The listing builds one solid part. Answer for the finished solid, in the listing's coordinates (mm). A direction names the side the tool comes from. Coordinates: 2 decimals unless noted, no trailing zeros. Write each loop counter-clockwise with the first axis right and the second up, starting at its lowest first coordinate (ties: lowest second). Pieces come first, ordered by that corner, then holes. Notation, with made-up numbers: M 59.25,-18 L 74.25,-18 A25 ccw 74.25,14 Z; hole C 85,42 d2. An arc over 180 degrees is marked long. Answer as CSV lines item,"result".
```python
from build123d import *

# Parameters (mm, degrees)
SKETCH1_W           = 15.307395447
SKETCH1_H           = 3.175
BOSS_EXTRUDE1_DEPTH = 16.27
SKETCH3_R           = 15.307395447
BOSS_EXTRUDE2_DEPTH = 3.175
CUT_EXTRUDE1_DEPTH  = 23.62
FILLET1_R           = 0.42


with BuildPart() as part:
    # Sketch1 → Revolve1 (revolve)
    with BuildSketch(Plane.XZ):
        with Locations((7.653697724, 1.5875)):
            Rectangle(SKETCH1_W, SKETCH1_H)
    revolve(axis=Axis((0, 0, 3.175), (0, 0, -1)))

    # Sketch2 → Boss-Extrude1 (add)
    with BuildSketch(Plane.XY.offset(3.175)):
        with BuildLine():
            Line((1.563453637, -12.031235681), (1.477576398, -11.370385062))
            ThreePointArc((1.477576398, -11.370385062), (0, -10.072395447), (-1.477576398, -11.370385062))
            Line((-1.477576398, -11.370385062), (-1.563453637, -12.031235681))
            ThreePointArc((-1.563453637, -12.031235681), (-2.366912935, -11.899274871), (-3.159711751, -11.713720201))
            Line((-3.159711751, -11.713720201), (-2.986155391, -11.070310044))
            ThreePointArc((-2.986155391, -11.070310044), (-3.854538862, -9.305679997), (-5.716360575, -9.939422028))
            Line((-5.716360575, -9.939422028), (-6.048597381, -10.517104592))
            ThreePointArc((-6.048597381, -10.517104592), (-6.740397766, -10.087718139), (-7.401839667, -9.612897005))
            Line((-7.401839667, -9.612897005), (-6.995272092, -9.084880673))
            ThreePointArc((-6.995272092, -9.084880673), (-7.122259124, -7.122259124), (-9.084880673, -6.995272092))
            Line((-9.084880673, -6.995272092), (-9.612897005, -7.401839667))
            ThreePointArc((-9.612897005, -7.401839667), (-10.087718139, -6.740397766), (-10.517104592, -6.048597381))
            Line((-10.517104592, -6.048597381), (-9.939422028, -5.716360575))
            ThreePointArc((-9.939422028, -5.716360575), (-9.305679997, -3.854538862), (-11.070310044, -2.986155391))
            Line((-11.070310044, -2.986155391), (-11.713720201, -3.159711751))
            ThreePointArc((-11.713720201, -3.159711751), (-11.899274871, -2.366912935), (-12.031235681, -1.563453637))
            Line((-12.031235681, -1.563453637), (-11.370385062, -1.477576398))
            ThreePointArc((-11.370385062, -1.477576398), (-10.072395447, 0), (-11.370385062, 1.477576398))
            Line((-11.370385062, 1.477576398), (-12.031235681, 1.563453637))
            ThreePointArc((-12.031235681, 1.563453637), (-11.899274871, 2.366912935), (-11.713720201, 3.159711751))
            Line((-11.713720201, 3.159711751), (-11.070310044, 2.986155391))
            ThreePointArc((-11.070310044, 2.986155391), (-9.305679997, 3.854538862), (-9.939422028, 5.716360575))
            Line((-9.939422028, 5.716360575), (-10.517104592, 6.048597381))
            ThreePointArc((-10.517104592, 6.048597381), (-10.087718139, 6.740397766), (-9.612897005, 7.401839667))
            Line((-9.612897005, 7.401839667), (-9.084880673, 6.995272092))
            ThreePointArc((-9.084880673, 6.995272092), (-7.122259124, 7.122259124), (-6.995272092, 9.084880673))
            Line((-6.995272092, 9.084880673), (-7.401839667, 9.612897005))
            ThreePointArc((-7.401839667, 9.612897005), (-6.740397766, 10.087718139), (-6.048597381, 10.517104592))
            Line((-6.048597381, 10.517104592), (-5.716360575, 9.939422028))
            ThreePointArc((-5.716360575, 9.939422028), (-3.854538862, 9.305679997), (-2.986155391, 11.070310044))
            Line((-2.986155391, 11.070310044), (-3.159711751, 11.713720201))
            ThreePointArc((-3.159711751, 11.713720201), (-2.366912935, 11.899274871), (-1.563453637, 12.031235681))
            Line((-1.563453637, 12.031235681), (-1.477576398, 11.370385062))
            ThreePointArc((-1.477576398, 11.370385062), (0, 10.072395447), (1.477576398, 11.370385062))
            Line((1.477576398, 11.370385062), (1.563453637, 12.031235681))
            ThreePointArc((1.563453637, 12.031235681), (2.366912935, 11.899274871), (3.159711751, 11.713720201))
            Line((3.159711751, 11.713720201), (2.986155391, 11.070310044))
            ThreePointArc((2.986155391, 11.070310044), (3.854538862, 9.305679997), (5.716360575, 9.939422028))
            Line((5.716360575, 9.939422028), (6.048597381, 10.517104592))
            ThreePointArc((6.048597381, 10.517104592), (6.740397766, 10.087718139), (7.401839667, 9.612897005))
            Line((7.401839667, 9.612897005), (6.995272092, 9.084880673))
            ThreePointArc((6.995272092, 9.084880673), (7.122259124, 7.122259124), (9.084880673, 6.995272092))
            Line((9.084880673, 6.995272092), (9.612897005, 7.401839667))
            ThreePointArc((9.612897005, 7.401839667), (10.087718139, 6.740397766), (10.517104592, 6.048597381))
            Line((10.517104592, 6.048597381), (9.939422028, 5.716360575))
            ThreePointArc((9.939422028, 5.716360575), (9.305679997, 3.854538862), (11.070310044, 2.986155391))
            Line((11.070310044, 2.986155391), (11.713720201, 3.159711751))
            ThreePointArc((11.713720201, 3.159711751), (11.899274871, 2.366912935), (12.031235681, 1.563453637))
            Line((12.031235681, 1.563453637), (11.370385062, 1.477576398))
            ThreePointArc((11.370385062, 1.477576398), (10.072395447, 0), (11.370385062, -1.477576398))
            Line((11.370385062, -1.477576398), (12.031235681, -1.563453637))
            ThreePointArc((12.031235681, -1.563453637), (11.899274871, -2.366912935), (11.713720201, -3.159711751))
            Line((11.713720201, -3.159711751), (11.070310044, -2.986155391))
            ThreePointArc((11.070310044, -2.986155391), (9.305679997, -3.854538862), (9.939422028, -5.716360575))
            Line((9.939422028, -5.716360575), (10.517104592, -6.048597381))
            ThreePointArc((10.517104592, -6.048597381), (10.087718139, -6.740397766), (9.612897005, -7.401839667))
            Line((9.612897005, -7.401839667), (9.084880673, -6.995272092))
            ThreePointArc((9.084880673, -6.995272092), (7.122259124, -7.122259124), (6.995272092, -9.084880673))
            Line((6.995272092, -9.084880673), (7.401839667, -9.612897005))
            ThreePointArc((7.401839667, -9.612897005), (6.740397766, -10.087718139), (6.048597381, -10.517104592))
            Line((6.048597381, -10.517104592), (5.716360575, -9.939422028))
            ThreePointArc((5.716360575, -9.939422028), (3.854538862, -9.305679997), (2.986155391, -11.070310044))
            Line((2.986155391, -11.070310044), (3.159711751, -11.713720201))
            ThreePointArc((3.159711751, -11.713720201), (2.366912935, -11.899274871), (1.563453637, -12.031235681))
        make_face()
    extrude(amount=BOSS_EXTRUDE1_DEPTH)

    # Sketch3 → Boss-Extrude2 (add)
    with BuildSketch(Plane(origin=(0, 0, 19.445), x_dir=(-1, 0, 0), z_dir=(0, 0, -1))):
        Circle(SKETCH3_R)
    extrude(amount=-BOSS_EXTRUDE2_DEPTH)

    # Sketch4 → Cut-Extrude1 (cut, through all)
    with BuildSketch(Plane.XY.offset(22.62)):
        Polygon((-7.478995387, 0), (-3.739497694, -6.477), (3.739497694, -6.477), (7.478995387, 0), (3.739497694, 6.477), (-3.739497694, 6.477), align=None)
    extrude(amount=-CUT_EXTRUDE1_DEPTH, mode=Mode.SUBTRACT)

    # Fillet1
    fillet1_edges = [part.edges().sort_by_distance(p)[0] for p in [
        (1.563453637, -12.031235681, 11.31),
        (3.159711751, -11.713720201, 11.31),
        (6.048597381, -10.517104592, 11.31),
        (7.401839667, -9.612897005, 11.31),
        (9.612897005, -7.401839667, 11.31),
        (10.517104592, -6.048597381, 11.31),
        (11.713720201, -3.159711751, 11.31),
        (12.031235681, -1.563453637, 11.31),
        (12.031235681, 1.563453637, 11.31),
        (11.713720201, 3.159711751, 11.31),
        (10.517104592, 6.048597381, 11.31),
        (9.612897005, 7.401839667, 11.31),
        (7.401839667, 9.612897005, 11.31),
        (6.048597381, 10.517104592, 11.31),
        (3.159711751, 11.713720201, 11.31),
        (1.563453637, 12.031235681, 11.31),
        (-1.563453637, 12.031235681, 11.31),
        (-3.159711751, 11.713720201, 11.31),
        (-6.048597381, 10.517104592, 11.31),
        (-7.401839667, 9.612897005, 11.31),
        (-9.612897005, 7.401839667, 11.31),
        (-10.517104592, 6.048597381, 11.31),
        (-11.713720201, 3.159711751, 11.31),
        (-12.031235681, 1.563453637, 11.31),
        (-12.031235681, -1.563453637, 11.31),
        (-11.713720201, -3.159711751, 11.31),
        (-10.517104592, -6.048597381, 11.31),
        (-9.612897005, -7.401839667, 11.31),
        (-7.401839667, -9.612897005, 11.31),
        (-6.048597381, -10.517104592, 11.31),
        (-3.159711751, -11.713720201, 11.31),
        (-1.563453637, -12.031235681, 11.31),
    ]]
    fillet(fillet1_edges, radius=FILLET1_R)


solid = part.part
```
Q1. Find section A-A (z = 1.5). Give the vertices of the cut face in (x, y), and give its area (3 significant figures).
Output:
outline,"C 0,0 d30.61; hole M -7.48,0 L -3.74,-6.48 L 3.74,-6.48 L 7.48,0 L 3.74,6.48 L -3.74,6.48 Z"
area,"591 mm2"
Q2. For faces 5 (the flat face through (-5.583, 3.284, 11.468)), 6 (the cylindrical face through (0.03, -10.073, 11.196)), 7 (the cylindrical face through (3.882, -9.294, 11.196)), 8 (the cylindrical face through (10.073, 0.03, 11.196)), 9 (the cylindrical face through (-0.03, 10.073, 11.196)), determine the directions among +Z, -Z, +X, -X, +Y, -Y from which every point of the face is accessible in a straight line to the end or side of a thin tool.
Output:
face 5,"+Z, -Z"
face 6,"-Y"
face 7,"none"
face 8,"+X"
face 9,"+Y"
Q3. Flat-ended cylindrical pins translate along their axes: pin 1 Ø1.5 at (y, z) = (3, 10.5) entering from +X; pin 2 Ø3 at (y, z) = (-4, 4.5) entering from -X; pin 3 Ø1.5 at (y, z) = (-8.5, 16) entering from -X. Find the tip coordinate at first contact, or state that the pin passes through.
Output:
pin 1,"x = 11.92"
pin 2,"x = -14.95"
pin 3,"x = -7.12"
Q4. Find section B-B (x = 0). Give the vertices of the cut face in (y, z) (3 decimals).
Output:
outline,"M -15.307,0 L -6.477,0 L -6.477,22.62 L -15.307,22.62 L -15.307,19.445 L -10.072,19.445 L -10.072,3.175 L -15.307,3.175 Z; M 6.477,0 L 15.307,0 L 15.307,3.175 L 10.072,3.175 L 10.072,19.445 L 15.307,19.445 L 15.307,22.62 L 6.477,22.62 Z"
Q5. The mould has two halves that part along Z. Classify faces 1 (the cylindrical face through (-10.073, -0.03, 11.196)), 2 (the flat face through (0.2, 10.4, 19.445)), 3 (the flat face through (0, 7, 0)), 4 (the flat face through (-5.635, -3.193, 11.468)): pulls with the +Z half, pulls with the -Z half, needs draft (parallel to the pull), parting line crosses it, or undercut.
Output:
face 1,"undercut"
face 2,"undercut"
face 3,"pulls with the -Z half"
face 4,"needs draft"
Q6. Find section C-C (y = -8.5). Give the vertices of the cut face in (x, z) (3 decimals).
Output:
outline,"M -12.731,0 L 12.731,0 L 12.731,3.175 L 6.722,3.175 L 6.722,19.445 L 12.731,19.445 L 12.731,22.62 L -12.731,22.62 L -12.731,19.445 L -6.722,19.445 L -6.722,3.175 L -12.731,3.175 Z"
Q7. Straight lines are drawn through the part: line 1 (X direction, y = 9.5, z = 13.5); line 2 (Z direction, x = -5.5, y = -11) (3 decimals); line 3 (X direction, y = -10, z = 17.5). For each, find the intervals that lie inside material, in ascending order.
Output:
line 1,"-7.23 to -5.33, -3.52 to 3.52, 5.33 to 7.23"
line 2,"0 to 3.175, 19.445 to 22.62"
line 3,"-6.87 to -5.75, -3.1 to 3.1, 5.75 to 6.87"
